The listing builds one solid part. Answer for the finished solid, in the listing's coordinates (mm). A direction names the side the tool comes from. Round coordinates to 2 decimals unless told otherwise and drop trailing zeros. Order: outer loops, then holes, each group sorted by start corner. A loop starts at its lowest first (then second) coordinate and runs counter-clockwise, first axis right, second up. Notation, with made-up numbers: (12.25, 60) - (51.25, 60) arc R21 cw to (51.25, 99) - close; hole circle Ø8 at (76, 41). An arc over 180 degrees is marked (long way). One line per item, written item: value. Start each with the question number.
1. Section C-C, the plane y = 4.5 is taken. Give the vertices of the cut face in (x, z).
2. Straight lines are drawn through the part: line 1 (X direction, y = 15, z = -15.5); line 2 (Z direction, x = -15, y = 17). For each, find the intervals that lie inside material, in ascending order.
3. Section A-A, the plane z = 0 is taken. Give the vertices of the cut face in (x, y).
4. For a pull along X with two mould halves and no side action, classify faces 3 (the flat face through (18.3, -1.3, -18.2)), 4 (the flat face through (-2, 34, 0)), 5 (the flat face through (15, 11.5, -16)) as released by +X, released by -X, zero draft, split by the parting line, or undercut.
5. Flat-ended cylindrical pins translate along their axes: P1, Ø2.5, axis at x = 15, z = 16, coming from the +Y side; P2, Ø0.9, axis at x = -15.5, z = 16, coming from the +Y side; P3, Ø17.5, axis at x = 3.5, z = -2, coming from the +Y side; P4, Ø1.5, axis at x = -5, z = 3.5, coming from the +Y side. Find the tip coordinate at first contact, or state that the pin passes through.
6. Section B-B, the plane x = 0 is taken. Give the vertices of the cut face in (y, z).
7. Section D-D, the plane z = 6 is taken. Give the vertices of the cut face in (x, y).
8. A tool of negligible diameter and unlimited length cuts with its end or side. For faces 1 (the cylindrical face through (-2.38, 20.49, 10.74)), 2 (the flat face through (-18.3, -1.3, 18.2)), from which of +Z, -Z, +X, -X, +Y, -Y can it reach the whole face along a straight path? Write none if from no direction.
from build123d import *

# Parameters (mm, degrees)
BOSS_EXTRUDE1_DEPTH = 11.5
BOSS_EXTRUDE2_DEPTH = 10
SKETCH4_R           = 1.5
BOSS_EXTRUDE3_DEPTH = 8
SKETCH5_R           = 11
BOSS_EXTRUDE4_DEPTH = 2
SKETCH6_R           = 2.5
BOSS_EXTRUDE5_DEPTH = 21
CUT_EXTRUDE1_DEPTH  = 18


with BuildPart() as part:
    # Sketch1 → Boss-Extrude1 (new body, symmetric)
    with BuildSketch(Plane(origin=(0, 0, 0), x_dir=(1, 0, 0), z_dir=(0, 1, 0))):
        Polygon((-15.5, -21), (15.5, -21), (21, -15.5), (21, 15.5), (15.5, 21), (-15.5, 21), (-21, 15.5), (-21, -15.5), align=None)
    extrude(amount=BOSS_EXTRUDE1_DEPTH, both=True)

    # Sketch3 → Boss-Extrude2 (add)
    with BuildSketch(Plane.XZ.offset(11.5)):
        Polygon((15.5, 21), (-15.5, 21), (-21, 15.5), (-21, -15.5), (-15.5, -21), (15.5, -21), (21, -15.5), (21, 15.5), align=None)
    extrude(amount=BOSS_EXTRUDE2_DEPTH)

    # Sketch4 → Boss-Extrude3 (add)
    with BuildSketch(Plane(origin=(0, 11.5, 0), x_dir=(1, 0, 0), z_dir=(0, 1, 0))):
        Polygon((-15.5, -21), (15.5, -21), (21, -15.5), (21, 15.5), (15.5, 21), (-15.5, 21), (-21, 15.5), (-21, -15.5), align=None)
        with Locations((-15.5, 15.5)):
            Circle(SKETCH4_R, mode=Mode.SUBTRACT)
        with Locations((15.5, 15.5)):
            Circle(SKETCH4_R, mode=Mode.SUBTRACT)
        with Locations((-15.5, -15.5)):
            Circle(SKETCH4_R, mode=Mode.SUBTRACT)
        with Locations((15.5, -15.5)):
            Circle(SKETCH4_R, mode=Mode.SUBTRACT)
    extrude(amount=BOSS_EXTRUDE3_DEPTH)

    # Sketch5 → Boss-Extrude4 (add)
    with BuildSketch(Plane(origin=(0, 19.5, 0), x_dir=(1, 0, 0), z_dir=(0, 1, 0))):
        Circle(SKETCH5_R)
    extrude(amount=BOSS_EXTRUDE4_DEPTH)

    # Sketch6 → Boss-Extrude5 (add)
    with BuildSketch(Plane(origin=(0, 21.5, 0), x_dir=(1, 0, 0), z_dir=(0, 1, 0))):
        Circle(SKETCH6_R)
    extrude(amount=BOSS_EXTRUDE5_DEPTH)

    # Sketch9 → Cut-Extrude1 (cut)
    with BuildSketch(Plane(origin=(0, 42.5, 0), x_dir=(1, 0, 0), z_dir=(0, 1, 0))):
        with BuildLine():
            Line((-2, 1.5), (-2, -1.5))
            ThreePointArc((-2, -1.5), (-2.5, 0), (-2, 1.5))
        make_face()
    extrude(amount=-CUT_EXTRUDE1_DEPTH, mode=Mode.SUBTRACT)


solid = part.part
Answer list:
1. outline: (-21, -15.5) - (-15.5, -21) - (15.5, -21) - (21, -15.5) - (21, 15.5) - (15.5, 21) - (-15.5, 21) - (-21, 15.5) - close
2. line 1: x = -21 to -17, -14 to 14, 17 to 21
2. line 2: z = -21 to -16.91, -14.09 to 14.09, 16.91 to 21
3. outline: (-21, -21.5) - (21, -21.5) - (21, 19.5) - (11, 19.5) - (11, 21.5) - (2.5, 21.5) - (2.5, 42.5) - (-2, 42.5) - (-2, 24.5) - (-2.5, 24.5) - (-2.5, 21.5) - (-11, 21.5) - (-11, 19.5) - (-21, 19.5) - close
4. face 3: released by +X
4. face 4: released by -X
4. face 5: undercut
5. P1: stops at y = 19.5
5. P2: stops at y = 11.5
5. P3: stops at y = 42.5
5. P4: stops at y = 21.5
6. outline: (-21.5, -21) - (19.5, -21) - (19.5, -11) - (21.5, -11) - (21.5, -2.5) - (42.5, -2.5) - (42.5, 2.5) - (21.5, 2.5) - (21.5, 11) - (19.5, 11) - (19.5, 21) - (-21.5, 21) - close
7. outline: (-21, -21.5) - (21, -21.5) - (21, 19.5) - (9.22, 19.5) - (9.22, 21.5) - (-9.22, 21.5) - (-9.22, 19.5) - (-21, 19.5) - close
8. face 1: +Y
8. face 2: +Z, -X, +Y, -Y
